The model under review builds one solid part; all positions refer to its coordinate system, in mm. Give positions to 0.01 mm unless a question says otherwise; leave off trailing zeros. Write each loop counter-clockwise with the first axis right and the second up, starting at its lowest first coordinate (ties: lowest second). Pieces come first, ordered by that corner, then holes. Notation, with made-up numbers: M 14.5,51.5 L 25.5,51.5 A12 cw 25.5,56.5 Z; hole C 75.5,72 d2. An arc over 180 degrees is marked long. Write item = value, one per line. Start each with the question number.
```python
from build123d import *

# Parameters (mm, degrees)
SKETCH1_W           = 1
SKETCH1_H           = 6
BOSS_EXTRUDE1_DEPTH = 2


with BuildPart() as part:
    # Sketch1 → Boss-Extrude1 (new body)
    with BuildSketch(Plane(origin=(0, 0, 0), x_dir=(0, 0, -1), z_dir=(1, 0, 0))):
        with BuildLine():
            Line((-18, 0), (-15, 0))
            Line((-15, 0), (-15, 2))
            Line((-15, 2), (-5, 2))
            Line((-5, 2), (-5, 0))
            Line((-5, 0), (5, 0))
            Line((5, 0), (5, 2))
            Line((5, 2), (15, 2))
            Line((15, 2), (15, 0))
            Line((15, 0), (18, 0))
            Line((18, 0), (18, -2))
            Line((18, -2), (22, -2))
            ThreePointArc((22, -2), (22.707106781, -2.292893219), (23, -3))
            Line((23, -3), (23, -11))
            ThreePointArc((23, -11), (22.707106781, -11.707106781), (22, -12))
            Line((22, -12), (18, -12))
            Line((18, -12), (18, -15))
            ThreePointArc((18, -15), (0, -11.536096634), (-18, -15))
            Line((-18, -15), (-18, -12))
            Line((-18, -12), (-22, -12))
            ThreePointArc((-22, -12), (-22.707106781, -11.707106781), (-23, -11))
            Line((-23, -11), (-23, -3))
            ThreePointArc((-23, -3), (-22.707106781, -2.292893219), (-22, -2))
            Line((-22, -2), (-18, -2))
            Line((-18, -2), (-18, 0))
        make_face()
        with BuildLine():
            Line((-15, -12.339136563), (-15, -6))
            ThreePointArc((-15, -6), (-14.121320344, -3.878679656), (-12, -3))
            Line((-12, -3), (12, -3))
            ThreePointArc((12, -3), (14.121320344, -3.878679656), (15, -6))
            Line((15, -6), (15, -12.339136563))
            ThreePointArc((15, -12.339136563), (0, -10.036096634), (-15, -12.339136563))
        make_face(mode=Mode.SUBTRACT)
        with Locations((-20.5, -7)):
            Rectangle(SKETCH1_W, SKETCH1_H, mode=Mode.SUBTRACT)
        with Locations((20.5, -7)):
            Rectangle(SKETCH1_W, SKETCH1_H, mode=Mode.SUBTRACT)
    extrude(amount=BOSS_EXTRUDE1_DEPTH)


solid = part.part
```
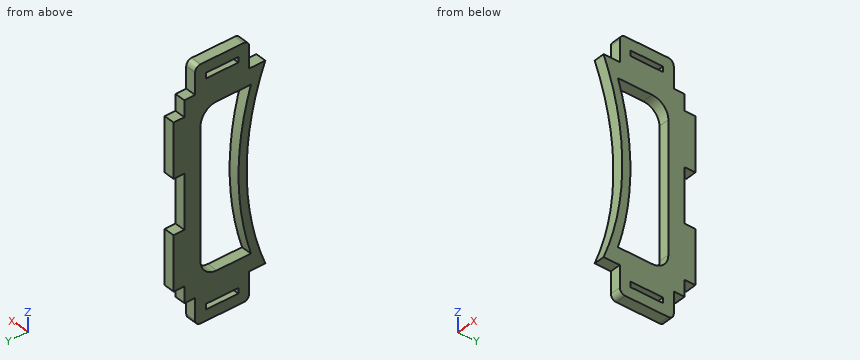
Item 1: We need section B-B, the plane x = 0.6. Give the number of separate pieces and of enclosed holes in the cut face, and give its area (3 significant figures).
Item 2: We need section A-A, the plane z = -3.5. Write out the cut boundary in (x, y), and give its area (3 significant figures).
Item 3: We need section C-C, the plane z = 4.5. Write out the cut boundary in (x, y), and give its area (3 significant figures).
Item 4: Clearance check with flat-ended pins moving along their axes: P1, Ø1.1, axis at x = 0.5, z = 20.5, coming from the +Y side; P2, Ø1, axis at x = 1, y = -13.5, coming from the +Z side; P3, Ø0.6, axis at x = 1.5, z = -16.5, coming from the +Y side. State where each tip first meets the part, or that it passes through.
Item 5: To check wall thickness, follow probe 1 along Z at (x, y) = (1.35, -9.75); probe 2 along Y at (x, z) = (1.6, -0.5); probe 3 along Z at (x, y) = (1.35, 0.75). State the ranges of each line that lie inside material, in increasing order. Write a range as [from, to].
Item 6: We need section D-D, the plane y = -1.25. Write out the cut boundary in (x, z), and give its area (3 significant figures).
Worked out:
q1.separate_pieces = 1
q1.enclosed_holes = 3
q1.area = 353 mm²
q2.outline = M 0,-11.66 L 2,-11.66 L 2,-10.16 L 0,-10.16 Z; M 0,-3 L 2,-3 L 2,0 L 0,0 Z
q2.area = 9.01 mm²
q3.outline = M 0,-11.75 L 2,-11.75 L 2,-10.24 L 0,-10.24 Z; M 0,-3 L 2,-3 L 2,0 L 0,0 Z
q3.area = 9.01 mm²
q4.P1 = -2
q4.P2 = 18
q4.P3 = 0
q5.probe_1 = [-23, -21], [-20, -15], [15, 20], [21, 23]
q5.probe_2 = [-11.54, -10.04], [-3, 0]
q5.probe_3 = [-15, -5], [5, 15]
q6.outline = M 0,-18 L 2,-18 L 2,18 L 0,18 Z
q6.area = 72.0 mm²
